from build123d import *

# Parameters (mm, degrees)
SKETCH_1_W          = 20
SKETCH_1_H          = 20
SKETCH_1_W_2        = 17
SKETCH_1_H_2        = 17
EXTRUDE_1_DEPTH     = 342.12
SKETCH_2_R          = 1.5
CUT_EXTRUDE_1_DEPTH = 343.84995902
SKETCH_3_R          = 1.5
CUT_EXTRUDE_2_DEPTH = 343.84995902


with BuildPart() as part:
    # 草图1 → 凸台-拉伸1 (new body)
    with BuildSketch(Plane.XY):
        Rectangle(SKETCH_1_W, SKETCH_1_H)
        Rectangle(SKETCH_1_W_2, SKETCH_1_H_2, mode=Mode.SUBTRACT)
    extrude(amount=EXTRUDE_1_DEPTH)

    # 草图2 → 切除-拉伸1 (cut, through all)
    with BuildSketch(Plane(origin=(0, 10, 0), x_dir=(1, 0, 0), z_dir=(0, 1, 0))):
        with Locations(Location((0, -5, 0), (0, 0, 270))):
            Circle(SKETCH_2_R)
        with Locations(Location((0, -20, 0), (0, 0, 270))):
            Circle(SKETCH_2_R)
        with Locations(Location((0, -337.12, 0), (0, 0, 270))):
            Circle(SKETCH_2_R)
        with Locations(Location((0, -322.12, 0), (0, 0, 270))):
            Circle(SKETCH_2_R)
    extrude(amount=-CUT_EXTRUDE_1_DEPTH, mode=Mode.SUBTRACT)

    # 草图3 → 切除-拉伸2 (cut, through all)
    with BuildSketch(Plane(origin=(0, 10, 0), x_dir=(1, 0, 0), z_dir=(0, 1, 0))):
        with Locations(Location((0, -35, 0), (0, 0, 270))):
            Circle(SKETCH_3_R)
        with Locations(Location((0, -50, 0), (0, 0, 270))):
            Circle(SKETCH_3_R)
        with Locations(Location((0, -65, 0), (0, 0, 270))):
            Circle(SKETCH_3_R)
        with Locations(Location((0, -80, 0), (0, 0, 270))):
            Circle(SKETCH_3_R)
        with Locations(Location((0, -95, 0), (0, 0, 270))):
            Circle(SKETCH_3_R)
        with Locations(Location((0, -110, 0), (0, 0, 270))):
            Circle(SKETCH_3_R)
        with Locations(Location((0, -125, 0), (0, 0, 270))):
            Circle(SKETCH_3_R)
        with Locations(Location((0, -140, 0), (0, 0, 270))):
            Circle(SKETCH_3_R)
        with Locations(Location((0, -155, 0), (0, 0, 270))):
            Circle(SKETCH_3_R)
        with Locations(Location((0, -170, 0), (0, 0, 270))):
            Circle(SKETCH_3_R)
        with Locations(Location((0, -185, 0), (0, 0, 270))):
            Circle(SKETCH_3_R)
        with Locations(Location((0, -200, 0), (0, 0, 270))):
            Circle(SKETCH_3_R)
        with Locations(Location((0, -215, 0), (0, 0, 270))):
            Circle(SKETCH_3_R)
        with Locations(Location((0, -230, 0), (0, 0, 270))):
            Circle(SKETCH_3_R)
        with Locations(Location((0, -245, 0), (0, 0, 270))):
            Circle(SKETCH_3_R)
        with Locations(Location((0, -260, 0), (0, 0, 270))):
            Circle(SKETCH_3_R)
        with Locations(Location((0, -275, 0), (0, 0, 270))):
            Circle(SKETCH_3_R)
        with Locations(Location((0, -290, 0), (0, 0, 270))):
            Circle(SKETCH_3_R)
        with Locations(Location((0, -305, 0), (0, 0, 270))):
            Circle(SKETCH_3_R)
    extrude(amount=-CUT_EXTRUDE_2_DEPTH, mode=Mode.SUBTRACT)


solid = part.part
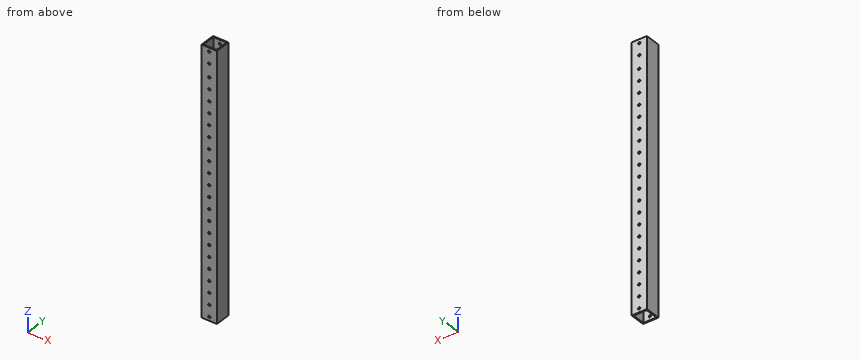
Design review of the part built by this model. Coordinates are the model's own, in mm. Coordinates: 2 decimals unless noted, no trailing zeros. Write each loop counter-clockwise with the first axis right and the second up, starting at its lowest first coordinate (ties: lowest second). Pieces come first, ordered by that corner, then holes. Notation, with made-up numbers: (-3.75, -12.75) - (6.25, -12.75) arc R13 ccw to (6.25, 12.25) - close; hole circle Ø3 at (63.5, -15). An arc over 180 degrees is marked (long way). One line per item, written item: value.
1) Add section C-C (z = 88). State the section outline as (x, y) points.
Answer sheet:
outline: (-10, -10) - (10, -10) - (10, 10) - (-10, 10) - close; hole (-8.5, -8.5) - (8.5, -8.5) - (8.5, 8.5) - (-8.5, 8.5) - close
2) Add section A-A (x = -5). State the section outline as (y, z) points.
Answer sheet:
outline: (-10, 0) - (-8.5, 0) - (-8.5, 342.12) - (-10, 342.12) - close; (8.5, 0) - (10, 0) - (10, 342.12) - (8.5, 342.12) - close
3) To check wall thickness, follow probe 1 along Y at (x, z) = (7.5, 17); probe 2 along X at (y, z) = (-9.4, 215). State the ranges of each line that lie inside material, in increasing order.
Answer sheet:
probe 1: y = -10 to -8.5, 8.5 to 10
probe 2: x = -10 to -1.5, 1.5 to 10
